```python
from build123d import *

# Parameters (mm, degrees)
SKETCH1_W                = 127
SKETCH1_H                = 76.2
BASE_EXTRUDE_DEPTH       = 44.45
SKETCH13_R               = 10.47242
CUT_EXTRUDE7_DEPTH       = 13.57122
CUT_EXTRUDE7_DRAFT       = -1.783333333
SKETCH14_R               = 8.9281
CUT_EXTRUDE8_DEPTH       = 114.3
SKETCH17_R               = 8.41883
CUT_EXTRUDE10_DEPTH      = 10.33018
CUT_EXTRUDE10_DRAFT      = -1.783333333
CUT_EXTRUDE11_REACH      = 182.583
CUT_EXTRUDE11_END_RADIUS = 8.9281
SKETCH18_R               = 7.3406
SKETCH21_R               = 8.41883
CUT_EXTRUDE13_DEPTH      = 10.33018
CUT_EXTRUDE13_DRAFT      = -1.783333333
CUT_EXTRUDE14_REACH      = 151.643
CUT_EXTRUDE14_END_RADIUS = 8.9281
SKETCH22_R               = 7.3406
SKETCH25_R               = 8.41883
CUT_EXTRUDE16_DEPTH      = 10.3378
CUT_EXTRUDE16_DRAFT      = -1.783333333
CUT_EXTRUDE17_REACH      = 124.053
CUT_EXTRUDE17_END_RADIUS = 8.9281
SKETCH26_R               = 7.3406
MIRROR1_COPY_1_SKETCH_R  = 8.41883
MIRROR1_COPY_1_DEPTH     = 10.33018
MIRROR1_COPY_1_DRAFT     = -1.783333333
MIRROR1_COPY_2_SKETCH_R  = 8.41883
MIRROR1_COPY_2_DEPTH     = 10.3378
MIRROR1_COPY_2_DRAFT     = -1.783333333
SKETCH29_R               = 5.1562
CUT_EXTRUDE19_DEPTH      = 87.36933773


with BuildPart() as part:
    # Sketch1 → Base-Extrude (new body)
    with BuildSketch(Plane.XY):
        Rectangle(SKETCH1_W, SKETCH1_H)
    extrude(amount=BASE_EXTRUDE_DEPTH)


with BuildPart() as cut_extrude7_tool:
    # Sketch13 → Cut-Extrude7 (with draft: the straight prism first)
    with BuildSketch(Plane(origin=(-63.5, 42.382338567, -29.074180248), x_dir=(0, 0, 1), z_dir=(-1, 0, 0))):
        with Locations((51.173800102, -42.382338567)):
            Circle(SKETCH13_R)
    extrude(amount=-CUT_EXTRUDE7_DEPTH)
    # Cut-Extrude7: the draft: its side faces are tilted about the plane it starts from
    cut_extrude7_sides = [cut_extrude7_tool.faces().sort_by_distance(p)[0] for p in [
        (-56.71439, 0, 11.627199854),
    ]]
    draft(cut_extrude7_sides, Plane(origin=(-63.5, 42.382338567, -29.074180248), x_dir=(0, 0, 1), z_dir=(-1, 0, 0)), CUT_EXTRUDE7_DRAFT)


with BuildPart() as part_1:
    add(part.part)

    # Cut-Extrude7: cut by cut_extrude7_tool
    add(cut_extrude7_tool.part, mode=Mode.SUBTRACT)

    # Sketch14 → Cut-Extrude8 (cut)
    with BuildSketch(Plane(origin=(-63.5, 38.1, -63.5), x_dir=(0, 0, 1), z_dir=(-1, 0, 0))):
        with Locations((85.599619854, -38.1)):
            Circle(SKETCH14_R)
    extrude(amount=-CUT_EXTRUDE8_DEPTH, mode=Mode.SUBTRACT)

    # Cut-Extrude9 cone 1 section (through the dimple's axis) → Cut-Extrude9 (revolve, cut)
    with BuildSketch(Plane(origin=(50.8, 0, 22.099619854), x_dir=(0, 0, 1), z_dir=(0, 1, 0))):
        Polygon((0, 0), (8.9281, 0), (0, 5.154640938), align=None)
    revolve(axis=Axis((50.8, 0, 22.099619854), (1, 0, 0)), mode=Mode.SUBTRACT)


with BuildPart() as cut_extrude10_tool:
    # Sketch17 → Cut-Extrude10 (with draft: the straight prism first)
    with BuildSketch(Plane(origin=(97.86363054, -38.1, 25.99710819), x_dir=(1, 0, 0), z_dir=(0, -1, 0))):
        with Locations((-59.76363054, -3.77210819)):
            Circle(SKETCH17_R)
    extrude(amount=-CUT_EXTRUDE10_DEPTH)
    # Cut-Extrude10: the draft: its side faces are tilted about the plane it starts from
    cut_extrude10_sides = [cut_extrude10_tool.faces().sort_by_distance(p)[0] for p in [
        (29.68117, -32.93491, 22.225),
    ]]
    draft(cut_extrude10_sides, Plane(origin=(97.86363054, -38.1, 25.99710819), x_dir=(1, 0, 0), z_dir=(0, -1, 0)), CUT_EXTRUDE10_DRAFT)


with BuildPart() as part_2:
    add(part_1.part)

    # Cut-Extrude10: cut by cut_extrude10_tool
    add(cut_extrude10_tool.part, mode=Mode.SUBTRACT)

    # Cut-Extrude11: up to this cylinder (the profile starts outside it)
    cut_extrude11_end = Plane(origin=(38.1, 0, 22.099619854), z_dir=(-1, 0, 0)) * Cylinder(CUT_EXTRUDE11_END_RADIUS, 384.0222, mode=Mode.PRIVATE)
    # Sketch18 → Cut-Extrude11 (cut, up to the surface)
    with BuildSketch(Plane(origin=(98.70252821, -38.1, 22.225), x_dir=(1, 0, 0), z_dir=(0, -1, 0)), mode=Mode.PRIVATE) as cut_extrude11_sk1:
        with Locations(Location((-60.60252821, 0, 0), (0, 0, 270))):
            Circle(SKETCH18_R)
    cut_extrude11_tool1 = extrude(cut_extrude11_sk1.sketch, amount=-CUT_EXTRUDE11_REACH, mode=Mode.PRIVATE) - cut_extrude11_end
    cut_extrude11 = cut_extrude11_tool1.solids().sort_by_distance((38.1, -38.1, 22.225))[0]
    add(cut_extrude11, mode=Mode.SUBTRACT)


with BuildPart() as cut_extrude13_tool:
    # Sketch21 → Cut-Extrude13 (with draft: the straight prism first)
    with BuildSketch(Plane(origin=(60.495960608, -38.1, 35.437611041), x_dir=(1, 0, 0), z_dir=(0, -1, 0))):
        with Locations((-60.495960608, -13.212611041)):
            Circle(SKETCH21_R)
    extrude(amount=-CUT_EXTRUDE13_DEPTH)
    # Cut-Extrude13: the draft: its side faces are tilted about the plane it starts from
    cut_extrude13_sides = [cut_extrude13_tool.faces().sort_by_distance(p)[0] for p in [
        (-8.41883, -32.93491, 22.225),
    ]]
    draft(cut_extrude13_sides, Plane(origin=(60.495960608, -38.1, 35.437611041), x_dir=(1, 0, 0), z_dir=(0, -1, 0)), CUT_EXTRUDE13_DRAFT)


with BuildPart() as part_3:
    add(part_2.part)

    # Cut-Extrude13: cut by cut_extrude13_tool
    add(cut_extrude13_tool.part, mode=Mode.SUBTRACT)

    # Cut-Extrude14: up to this cylinder (the profile starts outside it)
    cut_extrude14_end = Plane(origin=(0, 0, 22.099619854), z_dir=(-1, 0, 0)) * Cylinder(CUT_EXTRUDE14_END_RADIUS, 322.1422, mode=Mode.PRIVATE)
    # Sketch22 → Cut-Extrude14 (cut, up to the surface)
    with BuildSketch(Plane(origin=(61.334858278, -38.1, 31.665502851), x_dir=(1, 0, 0), z_dir=(0, -1, 0)), mode=Mode.PRIVATE) as cut_extrude14_sk1:
        with Locations(Location((-61.334858278, -9.440502851, 0), (0, 0, 270))):
            Circle(SKETCH22_R)
    cut_extrude14_tool1 = extrude(cut_extrude14_sk1.sketch, amount=-CUT_EXTRUDE14_REACH, mode=Mode.PRIVATE) - cut_extrude14_end
    add(cut_extrude14_tool1.solids().sort_by_distance((0, -38.1, 22.225))[0], mode=Mode.SUBTRACT)


with BuildPart() as cut_extrude16_tool:
    # Sketch25 → Cut-Extrude16 (with draft: the straight prism first)
    with BuildSketch(Plane(origin=(25.307359991, -38.1, 36.236677515), x_dir=(1, 0, 0), z_dir=(0, -1, 0))):
        with Locations((-63.407359991, -14.011677515)):
            Circle(SKETCH25_R)
    extrude(amount=-CUT_EXTRUDE16_DEPTH)
    # Cut-Extrude16: the draft: its side faces are tilted about the plane it starts from
    cut_extrude16_sides = [cut_extrude16_tool.faces().sort_by_distance(p)[0] for p in [
        (-46.51883, -32.9311, 22.225),
    ]]
    draft(cut_extrude16_sides, Plane(origin=(25.307359991, -38.1, 36.236677515), x_dir=(1, 0, 0), z_dir=(0, -1, 0)), CUT_EXTRUDE16_DRAFT)


with BuildPart() as part_4:
    add(part_3.part)

    # Cut-Extrude16: cut by cut_extrude16_tool
    add(cut_extrude16_tool.part, mode=Mode.SUBTRACT)

    # Cut-Extrude17: up to this cylinder (the profile starts outside it)
    cut_extrude17_end = Plane(origin=(-38.1, 0, 22.099619854), z_dir=(-1, 0, 0)) * Cylinder(CUT_EXTRUDE17_END_RADIUS, 266.9622, mode=Mode.PRIVATE)
    # Sketch26 → Cut-Extrude17 (cut, up to the surface)
    with BuildSketch(Plane(origin=(26.146257661, -38.1, 32.464569325), x_dir=(1, 0, 0), z_dir=(0, -1, 0)), mode=Mode.PRIVATE) as cut_extrude17_sk1:
        with Locations(Location((-64.246257661, -10.239569325, 0), (0, 0, 270))):
            Circle(SKETCH26_R)
    cut_extrude17_tool1 = extrude(cut_extrude17_sk1.sketch, amount=-CUT_EXTRUDE17_REACH, mode=Mode.PRIVATE) - cut_extrude17_end
    cut_extrude17 = cut_extrude17_tool1.solids().sort_by_distance((-38.1, -38.1, 22.225))[0]
    add(cut_extrude17, mode=Mode.SUBTRACT)

    # Mirror1: Cut-Extrude11, Cut-Extrude17 across plane
    add(cut_extrude11.mirror(Plane.ZX), mode=Mode.SUBTRACT)
    add(cut_extrude17.mirror(Plane.ZX), mode=Mode.SUBTRACT)


with BuildPart() as mirror1_copy_1_tool:
    # Mirror1 copy 1 sketch → Mirror1 copy 1 (with draft: the straight prism first)
    with BuildSketch(Plane(origin=(97.86363054, 38.1, 25.99710819), x_dir=(1, 0, 0), z_dir=(0, 1, 0))):
        with Locations((-59.76363054, 3.77210819)):
            Circle(MIRROR1_COPY_1_SKETCH_R)
    extrude(amount=-MIRROR1_COPY_1_DEPTH)
    # Mirror1 copy 1: the draft: its side faces are tilted about the plane it starts from
    mirror1_copy_1_sides = [mirror1_copy_1_tool.faces().sort_by_distance(p)[0] for p in [
        (29.68117, 32.93491, 22.225),
    ]]
    draft(mirror1_copy_1_sides, Plane(origin=(97.86363054, 38.1, 25.99710819), x_dir=(1, 0, 0), z_dir=(0, 1, 0)), MIRROR1_COPY_1_DRAFT)


with BuildPart() as part_5:
    add(part_4.part)

    # Mirror1 copy 1: cut by mirror1_copy_1_tool
    add(mirror1_copy_1_tool.part, mode=Mode.SUBTRACT)


with BuildPart() as mirror1_copy_2_tool:
    # Mirror1 copy 2 sketch → Mirror1 copy 2 (with draft: the straight prism first)
    with BuildSketch(Plane(origin=(25.307359991, 38.1, 36.236677515), x_dir=(1, 0, 0), z_dir=(0, 1, 0))):
        with Locations((-63.407359991, 14.011677515)):
            Circle(MIRROR1_COPY_2_SKETCH_R)
    extrude(amount=-MIRROR1_COPY_2_DEPTH)
    # Mirror1 copy 2: the draft: its side faces are tilted about the plane it starts from
    mirror1_copy_2_sides = [mirror1_copy_2_tool.faces().sort_by_distance(p)[0] for p in [
        (-46.51883, 32.9311, 22.225),
    ]]
    draft(mirror1_copy_2_sides, Plane(origin=(25.307359991, 38.1, 36.236677515), x_dir=(1, 0, 0), z_dir=(0, 1, 0)), MIRROR1_COPY_2_DRAFT)


with BuildPart() as part_6:
    add(part_5.part)

    # Mirror1 copy 2: cut by mirror1_copy_2_tool
    add(mirror1_copy_2_tool.part, mode=Mode.SUBTRACT)

    # Sketch29 → Cut-Extrude19 (cut, through all)
    with BuildSketch(Plane(origin=(0, 0, 0), x_dir=(-1, 0, 0), z_dir=(0, 0, -1))):
        with Locations((-19.05, -25.4)):
            Circle(SKETCH29_R)
        with Locations((19.05, 25.4)):
            Circle(SKETCH29_R)
    extrude(amount=-CUT_EXTRUDE19_DEPTH, mode=Mode.SUBTRACT)


solid = part_6.part
```
Could you check a few things on this model? Use its own coordinates, in mm. A direction names the side the tool comes from. Round coordinates to 2 decimals unless told otherwise and drop trailing zeros. Loops run counter-clockwise (first coordinate to the right, second up) from the corner with the lowest first, then second, coordinate; pieces in that order, holes last. Notation, with made-up numbers: (3, -17.75) -> (8, -17.75) arc R17 cw to (8, 14.25) -> close; hole circle Ø9 at (76.5, 82.25). An arc over 180 degrees is marked (long way). Put each result on its own line as item: value.
Q1. Thinking about a two-plate mould opening in X: for faces 1 (the flat face through (-63.5, 8, 12)), 2 (the flat face through (-1, 1, 44.45)), 3 (the cylindrical face through (40.3, -16.49, 15.22)), which applies, pulls with the +X half, pulls with the -X half, needs draft (parallel to the pull), parting line crosses it, or undercut?
Checks:
face 1: pulls with the -X half
face 2: needs draft
face 3: undercut
Q2. For pin 1 Ø13 at (x, z) = (42, 19.5) entering from -Y; pin 2 Ø9 at (x, z) = (0, 22.225) entering from -Y; pin 3 Ø10 at (y, z) = (1.5, 20.5) entering from -X, each with a flat end and sliding along its axis, tell me the tip position at first contact or that it passes through.
Checks:
pin 1: y = -38.1
pin 2: y = 7.64
pin 3: x = 51.8
Q3. I want a section at A-A on x = 19.05. Write out the boundary of the cut face in (y, z), and give its area (3 significant figures).
Checks:
outline: (-38.1, 0) -> (-30.56, 0) -> (-30.56, 44.45) -> (-38.1, 44.45) -> close; (-20.24, 0) -> (38.1, 0) -> (38.1, 44.45) -> (-20.24, 44.45) -> close; hole circle Ø17.86 at (0, 22.1)
area: 2,680 mm2
Q4. Which directions (+Z, -Z, +X, -X, +Y, -Y) give clear straight access to the entire face, cutting with the end or side of a thin tool? Please do faces 4 (the cylindrical face through (-0.269, 8.852, 20.937)), 5 (the conical face through (-44.655, 33.003, 27.251)), 6 (the cylindrical face through (40.3, 16.49, 15.22)), 7 (the cylindrical face through (-23.968, 26.949, 21.914)), 8 (the conical face through (-1.79, -33.01, 14.16)).
Checks:
face 4: -X
face 5: +Y
face 6: +Y, -Y
face 7: +Z, -Z
face 8: -Y
Q5. I want a section at C-C on z = 34.5. Write out the boundary of the cut face in (x, y), and give its area (3 significant figures).
Checks:
outline: (-63.5, -38.1) -> (63.5, -38.1) -> (63.5, 38.1) -> (-63.5, 38.1) -> close; hole circle Ø10.31 at (-19.05, 25.4); hole circle Ø10.31 at (19.05, -25.4)
area: 9,510 mm2
Q6. I want a section at D-D on x = -38.1. Write out the boundary of the cut face in (y, z), and give its area (3 significant figures).
Checks:
outline: (-38.1, 0) -> (38.1, 0) -> (38.1, 13.81) -> (27.76, 14.13) -> (27.76, 14.88) -> (5.26, 14.88) arc R8.93 cw to (-5.26, 14.88) -> (-27.76, 14.88) -> (-27.76, 14.13) -> (-38.1, 13.81) -> close; (-38.1, 30.64) -> (-27.76, 30.32) -> (-27.76, 29.57) -> (-4.9, 29.57) arc R8.93 cw to (4.9, 29.57) -> (27.76, 29.57) -> (27.76, 30.32) -> (38.1, 30.64) -> (38.1, 44.45) -> (-38.1, 44.45) -> close
area: 2,210 mm2
Q7. Please list where these lines run through material, in increasing order: line 1 (Y direction, x = 19, z = 33.5); line 2 (Z direction, x = -38.1, y = -13); line 3 (X direction, y = 27.5, z = 17.5). Write a range as from..to.
Checks:
line 1: -38.1..-30.56, -20.24..38.1
line 2: 0..14.88, 29.57..44.45
line 3: -63.5..-43.72, -32.48..-23.76, -14.34..32.48, 43.72..63.5
Q8. I want a section at B-B on y = -25.4. Write out the boundary of the cut face in (x, z) (3 decimals).
Checks:
outline: (-63.5, 0) -> (13.894, 0) -> (13.894, 44.45) -> (-63.5, 44.45) -> close; (24.206, 0) -> (63.5, 0) -> (63.5, 44.45) -> (24.206, 44.45) -> close; hole circle Ø14.681 at (-38.1, 22.225); hole circle Ø14.681 at (0, 22.225); hole circle Ø14.681 at (38.1, 22.225)
